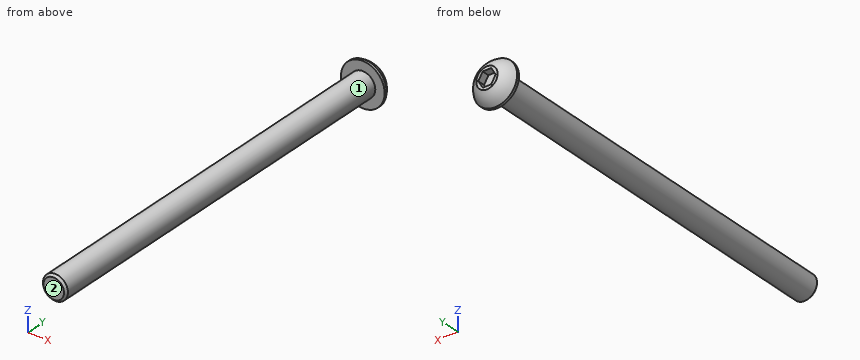
```python
from build123d import *

# Parameters (mm, degrees)
CUT_EXTRUDE1_DEPTH = 2.38125


with BuildPart() as part:
    # Sketch1 → Base-Revolve (revolve)
    with BuildSketch(Plane.XY):
        with BuildLine():
            Line((0, -127), (3.263194444, -127))
            Line((3.263194444, -127), (3.96875, -126.294444444))
            Line((3.96875, -126.294444444), (3.96875, 0))
            Line((3.96875, 0), (6.9469, 0))
            Line((6.9469, 0), (6.9469, 0.7874))
            ThreePointArc((6.9469, 0.7874), (5.442852348, 2.789756108), (3.384630657, 4.2164))
            Line((3.384630657, 4.2164), (0, 4.2164))
            Line((0, 4.2164), (0, -127))
        make_face()
    revolve(axis=Axis((0, 69.088, 0), (0, -1, 0)))

    # Sketch2 → Cut-Extrude1 (cut)
    with BuildSketch(Plane(origin=(0, 4.2164, 0), x_dir=(-1, 0, 0), z_dir=(0, 1, 0))):
        Polygon((-2.749630657, 0), (-1.374815329, -2.38125), (1.374815329, -2.38125), (2.749630657, 0), (1.374815329, 2.38125), (-1.374815329, 2.38125), align=None)
    extrude(amount=-CUT_EXTRUDE1_DEPTH, mode=Mode.SUBTRACT)


solid = part.part
```
Verification items for the finished model (mm, model axes). Face numbers are marked on the shaded views. A direction names the side the tool comes from. Give positions to 0.01 mm unless a question says otherwise; leave off trailing zeros. Order: outer loops, then holes, each group sorted by start corner. A loop starts at its lowest first (then second) coordinate and runs counter-clockwise, first axis right, second up. Notation, with made-up numbers: M 60,6 L 101,6 A22 ccw 101,38 Z; hole C 3.25,21.5 d5. An arc over 180 degrees is marked long. Return JSON: item names as keys, results as strings. Group by question number.
1) Go/stop test with flat-tipped pins: pin 1 Ø3 at (y, z) = (-92.5, -2.5) entering from -X; pin 2 Ø5 at (y, z) = (-68, 1) entering from +X; pin 3 Ø1.9 at (x, y) = (0, 3.5) entering from +Z. Record where each tip stops, or that it passes through.
2) Section check C-C on z = 5.5. Record the cut outline in (x, y), and give its area (3 significant figures).
3) Scan lines: line 1 (Y direction, x = 1, z = -1); line 2 (Z direction, x = 0.25, y = -95.5); line 3 (X direction, y = -104.5, z = 1.25). Record each from-to range of solid material in increasing order.
4) Section check A-A on x = 0. Record the cut outline in (y, z).
5) Access from +Z, -Z, +X, -X, +Y, -Y to the whole of each face (thin tool, end or side, straight path). Record for the marked faces 1 and 2.
6) Section check B-B on y = -47. Record the cut outline in (x, z).
Answer block:
{
 "1": {"pin 1": "stops at x = -3.84", "pin 2": "stops at x = 3.97", "pin 3": "stops at z = 5.68"},
 "2": {"outline": "M -4.24,0 L 4.24,0 L 4.24,0.79 A5.6 ccw -4.24,0.79 Z", "area": "18.1 mm^2"},
 "3": {"line 1": "y = -127 to 1.84", "line 2": "z = -3.96 to 3.96", "line 3": "x = -3.77 to 3.77"},
 "4": {"outline": "M -127,-3.26 L -126.29,-3.97 L 0,-3.97 L 0,-6.95 L 0.79,-6.95 A7.85 ccw 4.22,-3.38 L 4.22,-2.38 L 1.84,-2.38 L 1.84,2.38 L 4.22,2.38 L 4.22,3.38 A7.85 ccw 0.79,6.95 L 0,6.95 L 0,3.97 L -126.29,3.97 L -127,3.26 Z"},
 "5": {"face 1": "-Y", "face 2": "+Z, -Z, +X, -X, -Y"},
 "6": {"outline": "C 0,0 d7.94"}
}
